Could you check a few things on this model? Use its own coordinates, in mm. A direction names the side the tool comes from. Coordinates: 2 decimals unless noted, no trailing zeros. Order: outer loops, then holes, each group sorted by start corner. A loop starts at its lowest first (then second) coordinate and runs counter-clockwise, first axis right, second up. Notation, with made-up numbers: (-27.75, 88.25) -> (-11.75, 88.25) arc R11 ccw to (-11.75, 108.25) -> close; hole circle Ø5 at (15.5, 36.5). An arc over 180 degrees is marked (long way). Put each result on its own line as item: value. Start each with the question number.
Q1. If we section it at B-B (y = 938): Please give me the cut outline in (x, z).
Q2. If we section it at A-A (x = 510.5): Please give me the cut outline in (y, z), and give its area (3 significant figures).
Q3. If we section it at D-D (z = 2): Count the separate pieces of the cut face and the enclosed holes in it, and give its area (3 significant figures).
Q4. We'd pull the mould along Y, two halves only. Please class faces 1 (the face through (317.24, 422.85, 3.13)), 2 (the face through (1096.74, 589.06, 3.13)), 3 (the face through (371.056, 1283.945, 3.131)), 4 (the face through (161.4, 99.29, 3.13)): +Y half, -Y half, draft (parallel to the pull), parting line (faces both ways), or undercut.
Q5. Will these pins go through, and if not, where does the flat tip stop? pin 1 (18 mm diameter, centred on x = 273.17, y = 278.19, fed in from -Z); pin 2 (3 mm diameter, centred on y = 590.5, z = 2.5, fed in from +X); pin 3 (3 mm diameter, centred on y = 271.5, z = 2, fed in from -X); pin 4 (1 mm diameter, centred on x = 1719.5, z = 1.5, fed in from -Y).
Q6. If we section it at C-C (y = 559): Please give me the cut outline in (x, z), and give its area (3 significant figures).
Q7. For faces 5 (the face through (1905.068, 259.716, 3.131)), 6 (the face through (1022.954, 725.462, 3.131)), 7 (the face through (778.3, 361.426, 3.131)), 8 (the face through (1099.3, 1584.12, 3.13)), 9 (the face through (104.24, 852.02, 3.13)), which set-ups out of +Z, -Z, +X, -X, +Y, -Y let a thin tool reach every point of the face, with its end or its side?
Q8. Please list where these lines run through material, in increasing order: line 1 along X through (y, z) = (560, 0.75); line 2 along X through (y, z) = (679, 0.5); line 3 along X through (y, z) = (721.5, 0.5).
from build123d import *

# Parameters (mm, degrees)
MODEL_R             = 11.1125
BOSS_EXTRUDE1_DEPTH = 6.35


with BuildPart() as part:
    # Model → Boss-Extrude1 (new body)
    with BuildSketch(Plane.XY):
        with BuildLine():
            Line((5.108110735, 194.314892531), (163.618010499, 97.941859293))
            Line((163.618010499, 97.941859293), (322.127910263, 1.568826055))
            ThreePointArc((322.127910263, 1.568826055), (333.89428898, 1.914633478), (338.370752597, 12.801714096))
            ThreePointArc((338.370752597, 12.801714096), (351.434447306, 88.848287087), (388.196442443, 156.688519227))
            ThreePointArc((388.196442443, 156.688519227), (408.690944842, 177.077381556), (430.088955815, 196.51588618))
            ThreePointArc((430.088955815, 196.51588618), (536.177956286, 271.113973278), (655.171731621, 322.6914107))
            ThreePointArc((655.171731621, 322.6914107), (780.029083347, 362.033385202), (902.029382318, 409.499965959))
            ThreePointArc((902.029382318, 409.499965959), (943.4927889, 422.476908859), (986.713439487, 426.903024))
            ThreePointArc((986.713439487, 426.903024), (1029.934090103, 422.476908864), (1071.397496712, 409.499965959))
            ThreePointArc((1071.397496712, 409.499965959), (1193.397795685, 362.033385202), (1318.255147412, 322.691410699))
            ThreePointArc((1318.255147412, 322.691410699), (1437.248922745, 271.113973277), (1543.337923214, 196.51588618))
            ThreePointArc((1543.337923214, 196.51588618), (1564.735934188, 177.077381556), (1585.230436587, 156.688519227))
            ThreePointArc((1585.230436587, 156.688519227), (1621.992431724, 88.848287087), (1635.056126433, 12.801714096))
            ThreePointArc((1635.056126433, 12.801714096), (1639.53259005, 1.914633478), (1651.298968767, 1.568826055))
            Line((1651.298968767, 1.568826055), (1809.808868531, 97.941859293))
            Line((1809.808868531, 97.941859293), (1968.318768295, 194.314892531))
            ThreePointArc((1968.318768295, 194.314892531), (1973.426883996, 204.920287614), (1965.821440542, 213.90496795))
            ThreePointArc((1965.821440542, 213.90496795), (1904.319104128, 260.501148039), (1861.008833141, 324.360069187))
            ThreePointArc((1861.008833141, 324.360069187), (1829.125136948, 479.534965955), (1836.498090618, 637.779897071))
            ThreePointArc((1836.498090618, 637.779897071), (1868.895348354, 849.044814678), (1878.445908783, 1062.565854661))
            ThreePointArc((1878.445908783, 1062.565854661), (1885.489759902, 1113.896449039), (1909.00192278, 1160.065962298))
            ThreePointArc((1909.00192278, 1160.065962298), (1909.937478003, 1165.173079083), (1908.384310543, 1170.127428311))
            ThreePointArc((1908.384310543, 1170.127428311), (1904.700614553, 1173.786429442), (1899.735930337, 1175.306237344))
            ThreePointArc((1899.735930337, 1175.306237344), (1847.925642431, 1175.680168978), (1799.112371696, 1193.049980658))
            ThreePointArc((1799.112371696, 1193.049980658), (1605.15200634, 1282.837643457), (1402.680125607, 1351.303585593))
            ThreePointArc((1402.680125607, 1351.303585593), (1283.68635027, 1402.881023015), (1177.597349797, 1477.479110114))
            ThreePointArc((1177.597349797, 1477.479110114), (1156.199338824, 1496.917614738), (1135.704836425, 1517.306477067))
            ThreePointArc((1135.704836425, 1517.306477067), (1098.942841288, 1585.146709207), (1085.879146579, 1661.193282198))
            ThreePointArc((1085.879146579, 1661.193282198), (1083.573474575, 1670.091826663), (1075.253069645, 1673.999649433))
            Line((1075.253069645, 1673.999649433), (987.410269122, 1673.999649433))
            Line((987.410269122, 1673.999649433), (986.016609907, 1673.999649433))
            Line((986.016609907, 1673.999649433), (898.173809384, 1673.999649433))
            ThreePointArc((898.173809384, 1673.999649433), (889.853404455, 1670.091826664), (887.54773245, 1661.193282198))
            ThreePointArc((887.54773245, 1661.193282198), (874.484037741, 1585.146709206), (837.722042605, 1517.306477067))
            ThreePointArc((837.722042605, 1517.306477067), (817.227540206, 1496.917614738), (795.829529232, 1477.479110114))
            ThreePointArc((795.829529232, 1477.479110114), (689.74052876, 1402.881023015), (570.746753423, 1351.303585593))
            ThreePointArc((570.746753423, 1351.303585593), (368.274872692, 1282.837643458), (174.314507337, 1193.04998066))
            ThreePointArc((174.314507337, 1193.04998066), (125.5012366, 1175.680168978), (73.690948693, 1175.306237344))
            ThreePointArc((73.690948693, 1175.306237344), (68.726264477, 1173.786429442), (65.042568486, 1170.127428311))
            ThreePointArc((65.042568486, 1170.127428311), (63.489401027, 1165.173079083), (64.42495625, 1160.065962298))
            ThreePointArc((64.42495625, 1160.065962298), (87.937119128, 1113.896449039), (94.980970247, 1062.565854661))
            ThreePointArc((94.980970247, 1062.565854661), (104.531530676, 849.044814678), (136.928788412, 637.779897071))
            ThreePointArc((136.928788412, 637.779897071), (144.301742082, 479.534965955), (112.418045889, 324.360069187))
            ThreePointArc((112.418045889, 324.360069187), (69.107774901, 260.501148039), (7.605438488, 213.90496795))
            ThreePointArc((7.605438488, 213.90496795), (-4.967e-06, 204.920287614), (5.108110735, 194.314892531))
        make_face()
        with Locations((203.802894797, 164.060426103)):
            Circle(MODEL_R, mode=Mode.SUBTRACT)
        with Locations((273.165559958, 278.186921443)):
            Circle(MODEL_R, mode=Mode.SUBTRACT)
        with Locations((1769.623984233, 164.060426103)):
            Circle(MODEL_R, mode=Mode.SUBTRACT)
        with Locations((1700.261319072, 278.186921443)):
            Circle(MODEL_R, mode=Mode.SUBTRACT)
        with Locations((986.713439515, 506.390428564)):
            Circle(MODEL_R, mode=Mode.SUBTRACT)
        with Locations((986.713439515, 676.157132765)):
            Circle(MODEL_R, mode=Mode.SUBTRACT)
        with Locations((295.723951941, 1029.874581844)):
            Circle(MODEL_R, mode=Mode.SUBTRACT)
        with Locations((181.78107034, 1099.151145215)):
            Circle(MODEL_R, mode=Mode.SUBTRACT)
        with BuildLine():
            Line((345.096905092, 396.320114284), (344.999404352, 396.379394127))
            ThreePointArc((344.999404352, 396.379394127), (316.936053956, 423.300977152), (302.89359528, 459.565734456))
            ThreePointArc((302.89359528, 459.565734456), (284.961704097, 549.837677781), (267.850648214, 640.268802068))
            ThreePointArc((267.850648214, 640.268802068), (340.626263773, 997.19517935), (616.781657489, 1234.747126388))
            ThreePointArc((616.781657489, 1234.747126388), (760.772078282, 1287.024528435), (911.280552404, 1315.544122787))
            ThreePointArc((911.280552404, 1315.544122787), (948.659010331, 1323.142774148), (986.713439625, 1325.740663802))
            ThreePointArc((986.713439625, 1325.740663802), (1024.767868806, 1323.142774133), (1062.146326623, 1315.544122787))
            ThreePointArc((1062.146326623, 1315.544122787), (1212.654800747, 1287.024528436), (1356.64522154, 1234.747126389))
            ThreePointArc((1356.64522154, 1234.747126389), (1632.800615257, 997.195179351), (1705.576230816, 640.268802068))
            ThreePointArc((1705.576230816, 640.268802068), (1688.465174933, 549.837677782), (1670.533283749, 459.565734456))
            ThreePointArc((1670.533283749, 459.565734456), (1656.490825211, 423.300977357), (1628.4274751, 396.379394384))
            Line((1628.4274751, 396.379394384), (1628.329973938, 396.320114284))
            ThreePointArc((1628.329973938, 396.320114284), (1609.378608682, 387.631389964), (1588.933978787, 383.54907642))
            ThreePointArc((1588.933978787, 383.54907642), (1570.665812577, 383.937789322), (1552.854893643, 388.018005146))
            ThreePointArc((1552.854893643, 388.018005146), (1385.349426739, 437.316504437), (1218.71849884, 489.49463532))
            ThreePointArc((1218.71849884, 489.49463532), (1198.339741351, 497.735086266), (1179.358454519, 508.821543715))
            ThreePointArc((1179.358454519, 508.821543715), (1095.776005774, 590.387750311), (1044.679373403, 695.403015663))
            ThreePointArc((1044.679373403, 695.403015663), (1022.521857597, 725.776812519), (986.713439515, 737.234571316))
            ThreePointArc((986.713439515, 737.234571316), (950.905021434, 725.776812519), (928.747505628, 695.403015664))
            ThreePointArc((928.747505628, 695.403015664), (877.650873256, 590.387750312), (794.068424511, 508.821543716))
            ThreePointArc((794.068424511, 508.821543716), (775.087137679, 497.735086266), (754.70838019, 489.49463532))
            ThreePointArc((754.70838019, 489.49463532), (588.077452291, 437.316504437), (420.571985387, 388.018005147))
            ThreePointArc((420.571985387, 388.018005147), (402.761066453, 383.937789322), (384.492900242, 383.54907642))
            ThreePointArc((384.492900242, 383.54907642), (364.048270348, 387.631389964), (345.096905092, 396.320114284))
        make_face(mode=Mode.SUBTRACT)
        with Locations((1677.702927089, 1029.874581844)):
            Circle(MODEL_R, mode=Mode.SUBTRACT)
        with Locations((1791.64580869, 1099.151145215)):
            Circle(MODEL_R, mode=Mode.SUBTRACT)
        with Locations((986.713439515, 1386.202197897)):
            Circle(MODEL_R, mode=Mode.SUBTRACT)
        with Locations((986.713439515, 1519.552197898)):
            Circle(MODEL_R, mode=Mode.SUBTRACT)
    extrude(amount=BOSS_EXTRUDE1_DEPTH)


solid = part.part
The answers:
1. outline: (97.76, 0) -> (310.43, 0) -> (310.43, 6.35) -> (97.76, 6.35) -> close; (1663, 0) -> (1875.67, 0) -> (1875.67, 6.35) -> (1663, 6.35) -> close
2. outline: (255.92, 0) -> (414.09, 0) -> (414.09, 6.35) -> (255.92, 6.35) -> close; (1178.35, 0) -> (1333.45, 0) -> (1333.45, 6.35) -> (1178.35, 6.35) -> close
2. area: 1,990 mm^2
3. separate pieces: 1
3. enclosed holes: 13
3. area: 974,000 mm^2
4. face 1: undercut
4. face 2: undercut
4. face 3: +Y half
4. face 4: -Y half
5. pin 1: through
5. pin 2: x = 1830.28
5. pin 3: x = 77.65
5. pin 4: y = 42.73
6. outline: (145.55, 0) -> (283.19, 0) -> (283.19, 6.35) -> (145.55, 6.35) -> close; (852.02, 0) -> (1121.41, 0) -> (1121.41, 6.35) -> (852.02, 6.35) -> close; (1690.24, 0) -> (1827.88, 0) -> (1827.88, 6.35) -> (1690.24, 6.35) -> close
6. area: 3,460 mm^2
7. face 5: +Z, -Z, +X
7. face 6: +Z, -Z
7. face 7: +Z, -Z, -Y
7. face 8: +Z, -Z, +X, +Y
7. face 9: +Z, -Z, -X
8. line 1: 145.5 to 283, 852.94 to 1120.49, 1690.43 to 1827.93
8. line 2: 128.77 to 264.2, 923.57 to 975.97, 997.46 to 1049.86, 1709.22 to 1844.65
8. line 3: 121.31 to 263.29, 945.63 to 1027.8, 1710.14 to 1852.12
